Read the model definition and answer for the solid it produces. Units are mm, in the model's axes. Face numbers are marked on the shaded views. A direction names the side the tool comes from. Give positions to 0.01 mm unless a question says otherwise; leave off trailing zeros. Write each loop counter-clockwise with the first axis right and the second up, starting at its lowest first coordinate (ties: lowest second). Pieces come first, ordered by that corner, then holes. Notation, with made-up numbers: (34, 44.5) -> (72, 44.5) arc R22 ccw to (72, 83.5) -> close; hole circle Ø10 at (35, 18). An arc over 180 degrees is marked (long way). Write item = value, one per line.
Autodesk Inventor part; units mm, degrees
ref_plane "YZ Plane" through (0, 0, 0) normal (1, 0, 0) x (0, 1, 0)
ref_plane "XZ Plane" through (0, 0, 0) normal (0, 1, 0) x (-1, 0, 0)
ref_plane "XY Plane" through (0, 0, 0) normal (0, 0, 1) x (1, 0, 0)
sketch "Sketch1" plane through (0, 0, 0) normal (1, 0, 0) x (0, 1, 0)
  circle A0 centre (31.6, -9.4) radius 3
  circle A1 centre (31.6, -49.4) radius 3
  circle A2 centre (6.6, -9.4) radius 3
  circle A3 centre (6.6, -49.4) radius 3
  line L0 (31.6, -9.4) -> (6.6, -9.4) construction
  line L1 (6.6, -9.4) -> (6.6, -49.4) construction
  line L2 (6.6, -49.4) -> (31.6, -49.4) construction
  line L3 (31.6, -49.4) -> (31.6, -9.4) construction
  line L4 (0, 0) -> (38.2, 0)
  line L5 (38.2, 0) -> (38.2, -58.8)
  line L6 (38.2, -58.8) -> (0, -58.8)
  line L7 (0, -58.8) -> (0, 0)
  point P0 (31.6, -29.4)
  point P1 (38.2, -29.4)
  point P2 (19.1, -49.4)
  point P3 (19.1, -58.8)
  dimension "d0" = 6
  dimension "d1" = 25
  dimension "d2" = 40
  dimension "d3" = 58.8
  dimension "d4" = 38.2
extrude "Extrusion1" add sketch "Sketch1" along normal blind 10
sketch "Sketch3" plane through (10, 0, 0) normal (1, 0, 0) x (0, 0, -1)
  line L0 (58.8, 38.2) -> (0, 38.2)
  line L1 (0, 38.2) -> (0, 186.2)
  line L2 (2, 188.2) -> (56.8, 188.2)
  line L3 (58.8, 186.2) -> (58.8, 38.2)
  arc A0 (2, 188.2) -> (0, 186.2) centre (2, 186.2) ccw
  arc A1 (58.8, 186.2) -> (56.8, 188.2) centre (56.8, 186.2) ccw
  line L4 (14.4, 174.2) -> (44.4, 174.2)
  line L5 (44.4, 174.2) -> (44.4, 144.2)
  line L6 (44.4, 144.2) -> (14.4, 144.2)
  line L7 (14.4, 144.2) -> (14.4, 174.2)
  line L8 (14.4, 84.2) -> (44.4, 84.2)
  line L9 (44.4, 84.2) -> (44.4, 54.2)
  line L10 (44.4, 54.2) -> (14.4, 54.2)
  line L11 (14.4, 54.2) -> (14.4, 84.2)
  point P0 (0, 0)
  point P1 (29.4, 38.2)
  point P2 (29.4, 174.2)
  point P3 (29.4, 84.2)
  point P4 (29.4, 188.2)
  point P5 (29.4, 38.2)
  point P6 (29.4, 54.2)
  point P7 (29.4, 38.2)
  dimension "d7" = 150
  dimension "d8" = 2
  dimension "d9" = 30
  dimension "d12" = 60
  dimension "d13" = 16
extrude "Extrusion2" add sketch "Sketch3" against normal blind 10
sketch "Sketch4" plane through (0, 0, 0) normal (-1, 0, 0) x (0, 0, 1)
  circle A0 centre (-52.97, 139.57) radius 3
  circle A1 centre (-5.83, 139.57) radius 3
  circle A2 centre (-52.97, 92.43) radius 3
  circle A3 centre (-5.83, 92.43) radius 3
  line L0 (-52.97, 92.43) -> (-5.83, 92.43) construction
  line L1 (-5.83, 92.43) -> (-5.83, 139.57) construction
  line L2 (-5.83, 139.57) -> (-52.97, 139.57) construction
  line L3 (-52.97, 139.57) -> (-52.97, 92.43) construction
  line L4 (-57.6, 87.8) -> (-1.2, 87.8) construction
  line L5 (-1.2, 87.8) -> (-1.2, 144.2) construction
  line L6 (-1.2, 144.2) -> (-57.6, 144.2) construction
  line L7 (-57.6, 144.2) -> (-57.6, 87.8) construction
  line L8 (-14.4, 144.2) -> (-44.4, 144.2) construction
  circle A4 centre (-29.4, 116) radius 17.5
  line L9 (-8.4, 116) -> (-29.4, 137) construction
  line L10 (-29.4, 137) -> (-50.4, 116) construction
  line L11 (-50.4, 116) -> (-29.4, 95) construction
  line L12 (-29.4, 95) -> (-8.4, 116) construction
  circle A5 centre (-29.4, 137) radius 2.25
  circle A6 centre (-50.4, 116) radius 2.25
  circle A7 centre (-8.4, 116) radius 2.25
  circle A8 centre (-29.4, 95) radius 2.25
  point P0 (0, 0)
  point P1 (-1.2, 116)
  point P2 (-5.83, 116)
  point P3 (-29.4, 139.57)
  point P4 (-29.4, 144.2)
  point P5 (-29.4, 144.2)
  dimension "d16" = 47.14
  dimension "d17" = 6
  dimension "d18" = 56.4
  dimension "d19" = 35
  dimension "d22" = 42
  dimension "d23" = 4.5
extrude "Extrusion3" cut sketch "Sketch4" against normal up to surface (10 mm away)
properties part number "Y_Gantry_Connector"
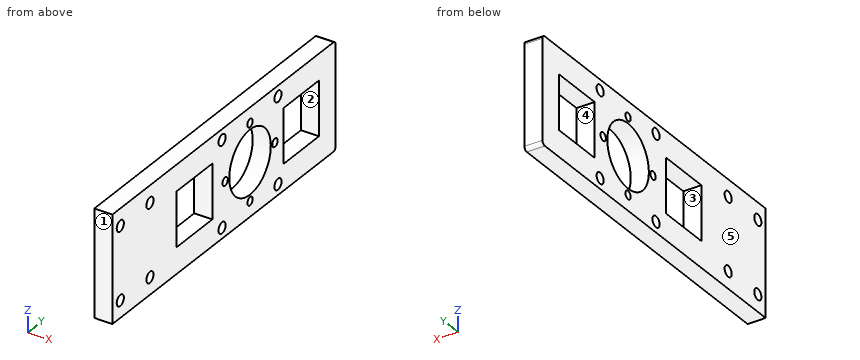
(1) The part is cut by section B-B on y = 116. Determine the outline of the cut face in (x, z), plus the area to 3 significant figures.
Checks:
outline = (0, -58.8) -> (10, -58.8) -> (10, -52.65) -> (0, -52.65) -> close; (0, -48.15) -> (10, -48.15) -> (10, -46.9) -> (0, -46.9) -> close; (0, -11.9) -> (10, -11.9) -> (10, -10.65) -> (0, -10.65) -> close; (0, -6.15) -> (10, -6.15) -> (10, 0) -> (0, 0) -> close
area = 148 mm²
(2) The part is cut by section A-A on y = 80.5. Determine the outline of the cut face in (x, z).
Checks:
outline = (0, -58.8) -> (10, -58.8) -> (10, -44.4) -> (0, -44.4) -> close; (0, -14.4) -> (10, -14.4) -> (10, 0) -> (0, 0) -> close
(3) A tool of negligible diameter and unlimited length cuts with its end or side. For the marked faces 1 and 2, from which of +Z, -Z, +X, -X, +Y, -Y can it reach the whole face along a straight path? Write none if from no direction.
Checks:
face_1 = +Z, -Z, +X, -X, -Y
face_2 = +X, -X
(4) The part is cut by section D-D on z = -29.4. Determine the outline of the cut face in (x, y), plus the area to 3 significant figures.
Checks:
outline = (0, 0) -> (10, 0) -> (10, 54.2) -> (0, 54.2) -> close; (0, 84.2) -> (10, 84.2) -> (10, 92.75) -> (0, 92.75) -> close; (0, 97.25) -> (10, 97.25) -> (10, 98.5) -> (0, 98.5) -> close; (0, 133.5) -> (10, 133.5) -> (10, 134.75) -> (0, 134.75) -> close; (0, 139.25) -> (10, 139.25) -> (10, 144.2) -> (0, 144.2) -> close; (0, 174.2) -> (10, 174.2) -> (10, 188.2) -> (0, 188.2) -> close
area = 842 mm²
(5) The part is cut by section C-C on x = 2. Count the separate pieces of the cut face and the enclosed holes in it, plus the area to 3 significant figures.
Checks:
separate_pieces = 1
enclosed_holes = 15
area = 8,010 mm²
(6) Consider L1, parallel to Z at x = 3, y = 139.57; L2, parallel to Y at x = 3.75, z = -53; L3, parallel to Y at x = 6, z = -29.4. Determine where each line is inside the solid, lowest interval first.
Checks:
L1 = -58.8 to -55.97, -49.97 to -8.83, -2.83 to 0
L2 = 0 to 89.43, 95.43 to 136.57, 142.57 to 188.2
L3 = 0 to 54.2, 84.2 to 92.75, 97.25 to 98.5, 133.5 to 134.75, 139.25 to 144.2, 174.2 to 188.2
(7) For a pull along Z with two mould halves and no side action, classify the marked faces 3, 4 and 5 as released by +Z, released by -Z, zero draft, split by the parting line, or undercut.
Checks:
face_3 = undercut
face_4 = undercut
face_5 = zero draft
(8) Given P1, Ø1.5, axis at y = 139, z = -6.5, coming from the -X side, flat-ended and moving along its own axis, determine where the tip first touches the part or whether it passes through.
Checks:
P1 = through
